Work out the finished part from the listing and answer in its coordinate system (mm). Face numbers are marked on the shaded views. A direction names the side the tool comes from. Coordinates: 2 decimals unless noted, no trailing zeros. Order: outer loops, then holes, each group sorted by start corner. A loop starts at its lowest first (then second) coordinate and runs counter-clockwise, first axis right, second up.
1. The part is cut by section A-A, the plane x = 16.3. Give the vertices of the cut face in (y, z), then the cut area to 3 significant figures.
2. Find the intervals of material crossed by probe 1 along Z at (x, y) = (-17.7, -3.3); probe 2 along Z at (x, y) = (15.5, -10.25); probe 3 along X at (y, z) = (-10, 1.25), in increasing order.
3. The part is cut by section B-B, the plane z = 0. Give the vertices of the cut face in (x, y).
4. Determine the mould class of the marked faces 3, 4 and 5 for opening direction Z: +Z half, -Z half, draft (parallel to the pull), parting line (faces both ways), or undercut.
5. A tool of negligible diameter and unlimited length cuts with its end or side. For the marked faces 1 and 2, from which of +Z, -Z, +X, -X, +Y, -Y can it reach the whole face along a straight path? Write none if from no direction.
6. The part is cut by section C-C, the plane y = -7. Give the vertices of the cut face in (x, z).
```python
from build123d import *

# Parameters (mm, degrees)
F0_W     = 50
F0_H     = 12
F1_DEPTH = 12
F2_W     = 44.2
F2_H     = 6.2
F3_DEPTH = 7
F4_R     = 1.35
F5_DEPTH = 5


with BuildPart() as f1:
    # F0 (on Front) → F1 (new body)
    with BuildSketch(Plane.XZ):
        Rectangle(F0_W, F0_H)
    extrude(amount=F1_DEPTH)

    # F2 (on face) → F3 (cut)
    with BuildSketch(Plane.XZ.offset(12)):
        Rectangle(F2_W, F2_H)
    extrude(amount=-F3_DEPTH, mode=Mode.SUBTRACT)

    # F4 (on face) → F5 (cut, through all)
    with BuildSketch(Plane.XZ.offset(5)):
        with Locations((-17.7, 0)):
            Circle(F4_R)
        with Locations((16.3, 0)):
            Circle(F4_R)
    extrude(amount=-F5_DEPTH, mode=Mode.SUBTRACT)


solid = f1.part
```
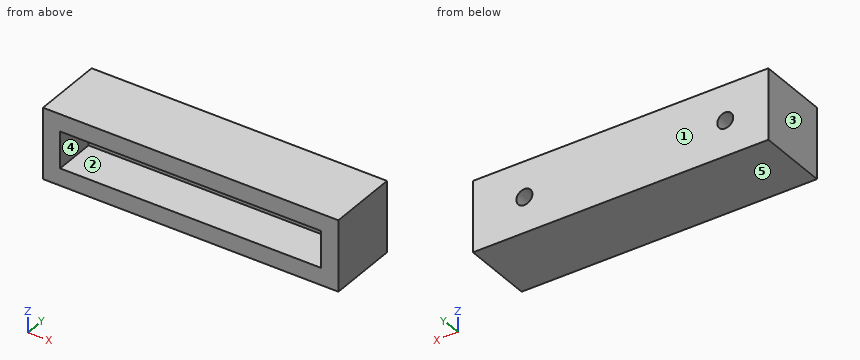
Geometry says:
1. outline: (-12, -6) - (0, -6) - (0, -1.35) - (-5, -1.35) - (-5, -3.1) - (-12, -3.1) - close; (-12, 3.1) - (-5, 3.1) - (-5, 1.35) - (0, 1.35) - (0, 6) - (-12, 6) - close
1. area: 87.1 mm2
2. probe 1: z = -6 to -1.35, 1.35 to 6
2. probe 2: z = -6 to -3.1, 3.1 to 6
2. probe 3: x = -25 to -22.1, 22.1 to 25
3. outline: (-25, -12) - (-22.1, -12) - (-22.1, -5) - (-19.05, -5) - (-19.05, 0) - (-25, 0) - close; (-16.35, -5) - (14.95, -5) - (14.95, 0) - (-16.35, 0) - close; (17.65, -5) - (22.1, -5) - (22.1, -12) - (25, -12) - (25, 0) - (17.65, 0) - close
4. face 3: draft
4. face 4: undercut
4. face 5: -Z half
5. face 1: +Z, -Z, +X, -X, +Y
5. face 2: -Y
6. outline: (-25, -6) - (25, -6) - (25, 6) - (-25, 6) - close; hole (-22.1, -3.1) - (22.1, -3.1) - (22.1, 3.1) - (-22.1, 3.1) - close
